For this review, take the finished solid that the model builds, in its own axes (mm). Face numbers are marked on the shaded views. Give positions to 0.01 mm unless a question says otherwise; leave off trailing zeros.
Q1. Mouldability with a two-part tool opening along X and no side actions: class the marked faces 1, 2, 3 and 4 as released by +X, released by -X, zero draft, split by the parting line, or undercut.
Q2. For line 1 (Z direction, x = 0.5, y = 4); line 2 (Y direction, x = 1, z = -1.5); line 3 (X direction, y = 3.5, z = 1), list the stretches that pass through material, from the lowest coordinate up.
Q3. Insertion check: P1, Ø3, axis at x = 0, z = 0, coming from the -Y side; P2, Ø3, axis at x = 4, y = 4.5, coming from the -Z side; P3, Ø1, axis at x = -1.5, y = 3.5, coming from the +Z side; P4, Ø0.8, axis at x = 1, y = 4.5, coming from the -Z side. Each pin has a flat end and moves straight along its axis. Give the tip position at first contact, or say it passes through.
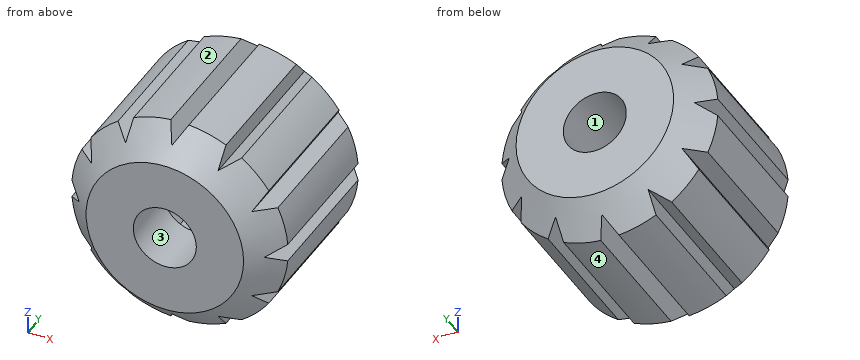
```python
from build123d import *

# Parameters (mm, degrees)
CUT_EXTRUDE1_DEPTH = 11
CUT_EXTRUDE2_DEPTH = 2.8


with BuildPart() as part:
    # Sketch1 → Revolve1 (revolve)
    with BuildSketch(Plane.XY):
        Polygon((1.6, 0), (4, 0), (5.5, 1.5), (5.5, 8.5), (4, 10), (1.6, 10), align=None)
    revolve(axis=Axis((0, 9.5, 0), (0, -1, 0)))

    # Sketch2 → Cut-Extrude1 (cut, through all)
    with BuildSketch(Plane(origin=(0, 10, 0), x_dir=(1, 0, 0), z_dir=(0, 1, 0))):
        Polygon((-0.849983323, 6.145149701), (0, 4.697880799), (0.849983323, 6.145149701), align=None)
        Polygon((3.808682001, 4.896864089), (2.3364677, 5.746847412), (2.3489404, 4.068484116), align=None)
        Polygon((5.746847412, 2.3364677), (4.896864089, 3.808682001), (4.068484116, 2.3489404), align=None)
        Polygon((6.145149701, -0.849983323), (6.145149701, 0.849983323), (4.697880799, 0), align=None)
        Polygon((4.896864089, -3.808682001), (5.746847412, -2.3364677), (4.068484116, -2.3489404), align=None)
        Polygon((2.3364677, -5.746847412), (3.808682001, -4.896864089), (2.3489404, -4.068484116), align=None)
        Polygon((-0.849983323, -6.145149701), (0.849983323, -6.145149701), (0, -4.697880799), align=None)
        Polygon((-3.808682001, -4.896864089), (-2.3364677, -5.746847412), (-2.3489404, -4.068484116), align=None)
        Polygon((-5.746847412, -2.3364677), (-4.896864089, -3.808682001), (-4.068484116, -2.3489404), align=None)
        Polygon((-6.145149701, 0.849983323), (-6.145149701, -0.849983323), (-4.697880799, 0), align=None)
        Polygon((-4.896864089, 3.808682001), (-5.746847412, 2.3364677), (-4.068484116, 2.3489404), align=None)
        Polygon((-2.3364677, 5.746847412), (-3.808682001, 4.896864089), (-2.3489404, 4.068484116), align=None)
    extrude(amount=-CUT_EXTRUDE1_DEPTH, mode=Mode.SUBTRACT)

    # Sketch3 → Cut-Extrude2 (cut)
    with BuildSketch(Plane(origin=(0, 3, 0), x_dir=(-1, 0, 0), z_dir=(0, -1, 0))):
        Polygon((1.674315781, 2.9), (-1.674315781, 2.9), (-3.348631561, 0), (-1.674315781, -2.9), (1.674315781, -2.9), (3.348631561, 0), align=None)
    extrude(amount=-CUT_EXTRUDE2_DEPTH, mode=Mode.SUBTRACT)


solid = part.part
```
Computed:
1. face 1: undercut
1. face 2: released by -X
1. face 3: undercut
1. face 4: released by +X
2. line 1: z = -5.48 to -2.9, 2.9 to 5.48
2. line 2: y = 0 to 3, 5.8 to 10
2. line 3: x = -5.41 to -2.77, 2.77 to 5.41
3. P1: passes through
3. P2: stops at z = -4.52
3. P3: stops at z = 5.41
3. P4: stops at z = -5.47
